The drawing under review shows one solid part. Ordinate dimensions are in mm from its lowest x, y, z. A direction names the side the tool comes from. Coordinates: 2 decimals unless noted, no trailing zeros. Order: outer loops, then holes, each group sorted by start corner. A loop starts at its lowest first (then second) coordinate and runs counter-clockwise, first axis right, second up. Notation, with made-up numbers: (-17.75, 71) - (33.25, 71) arc R34 cw to (33.25, 110) - close; hole circle Ø2 at (10, 71.5). An arc over 180 degrees is marked (long way). Answer in a Markdown table with one row per item.
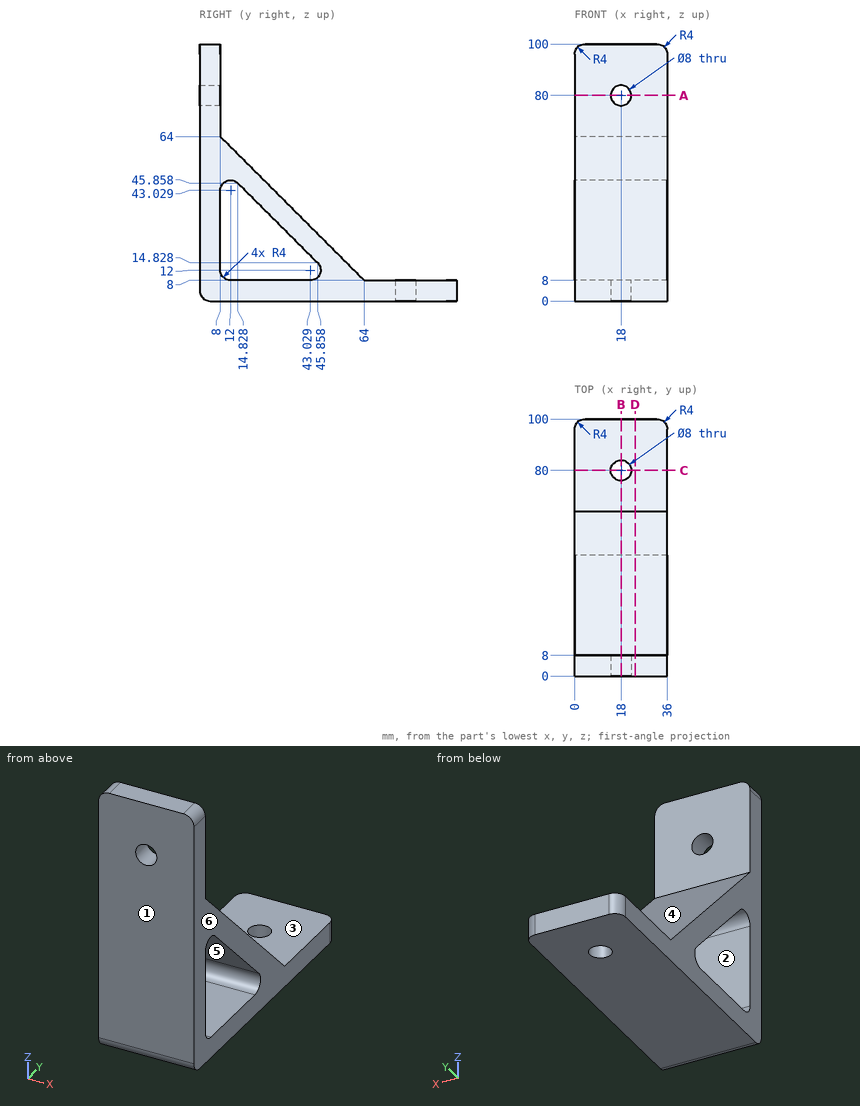
Item 1: Clearance check with flat-ended pins moving along their axes: pin 1 Ø11 at (x, z) = (12.5, 73.5) entering from +Y; pin 2 Ø15.5 at (x, y) = (13, 34) entering from +Z; pin 3 Ø10.5 at (x, y) = (18, 80) entering from +Z. State where each tip first meets the part, or that it passes through.
Check values:
| item | result |
|---|---|
| pin 1 | y = 8 |
| pin 2 | z = 45.75 |
| pin 3 | z = 8 |
Item 2: We need section A-A, the plane z = 80. Write out the cut boundary in (x, y).
Check values:
| item | result |
|---|---|
| outline | (0, 0) - (14, 0) - (14, 8) - (0, 8) - close; (22, 0) - (36, 0) - (36, 8) - (22, 8) - close |
Item 3: We need section D-D, the plane x = 23.5. Write out the cut boundary in (y, z).
Check values:
| item | result |
|---|---|
| outline | (0, 4) arc R4 ccw to (4, 0) - (100, 0) - (100, 8) - (64, 8) - (8, 64) - (8, 100) - (0, 100) - close; hole (8, 12) arc R4 ccw to (12, 8) - (43.03, 8) arc R4 ccw to (45.86, 14.83) - (14.83, 45.86) arc R4 ccw to (8, 43.03) - close |
Item 4: Tool access review of the marked faces 1, 2 and 3: name each direction out of +Z, -Z, +X, -X, +Y, -Y from which nothing blocks a thin tool from reaching the whole face with its end or side.
Check values:
| item | result |
|---|---|
| face 1 | +Z, -Z, +X, -X, -Y |
| face 2 | +X, -X |
| face 3 | +Z, +X, -X, +Y |
Item 5: We need section B-B, the plane x = 18. Write out the cut boundary in (y, z).
Check values:
| item | result |
|---|---|
| outline | (0, 4) arc R4 ccw to (4, 0) - (76, 0) - (76, 8) - (64, 8) - (8, 64) - (8, 76) - (0, 76) - close; (0, 84) - (8, 84) - (8, 100) - (0, 100) - close; (84, 0) - (100, 0) - (100, 8) - (84, 8) - close; hole (8, 12) arc R4 ccw to (12, 8) - (43.03, 8) arc R4 ccw to (45.86, 14.83) - (14.83, 45.86) arc R4 ccw to (8, 43.03) - close |
Item 6: To check wall thickness, follow line 1 (X direction, y = 80, z = 1.5); line 2 (Y direction, x = 6, z = 18) (1 decimal); line 3 (Y direction, x = 6.5, z = 37.5) (1 decimal). State the ranges of each line that lie inside material, in increasing order. Write a range as from..to.
Check values:
| item | result |
|---|---|
| line 1 | 0..14, 22..36 |
| line 2 | 0..8, 42.7..54 |
| line 3 | 0..8, 23.2..34.5 |
Item 7: Mouldability with a two-part tool opening along Z and no side actions: class the marked faces 4, 5 and 6 as +Z half, -Z half, draft (parallel to the pull), parting line (faces both ways), or undercut.
Check values:
| item | result |
|---|---|
| face 4 | +Z half |
| face 5 | undercut |
| face 6 | draft |
